Can you work these out from the model? Positions are in its coordinate system, mm. Face numbers are marked on the shaded views. A direction names the side the tool comes from. Round coordinates to 2 decimals unless told otherwise and drop trailing zeros. Order: outer loops, then holes, each group sorted by start corner. A loop starts at its lowest first (then second) coordinate and runs counter-clockwise, first axis right, second up. Notation, with made-up numbers: M 4.5,73 L 39.5,73 A23 ccw 39.5,100 Z; hole C -33,2 d11. An arc over 180 degrees is marked long. Answer as CSV lines item,"result". Start each with the question number.
from build123d import *

# Parameters (mm, degrees)
SKETCH1_R               = 50.8
BOSS_EXTRUDE1_DEPTH     = 101.6
CUT_EXTRUDE1_DEPTH      = 96.52
CUT_EXTRUDE1_DEPTH_BACK = 101.6
SKETCH2_R               = 6.35
CUT_EXTRUDE2_DEPTH      = 103.886
CUT_EXTRUDE2_DEPTH_BACK = 86.36
SKETCH3_W               = 76.2
SKETCH3_H               = 82.476489684


with BuildPart() as part:
    # Sketch1 → Boss-Extrude1 (new body)
    with BuildSketch(Plane(origin=(0, 0, 0), x_dir=(1, 0, 0), z_dir=(0, 1, 0))):
        with Locations(Location((0, 0, 0), (0, 0, 270))):
            Circle(SKETCH1_R)
    extrude(amount=BOSS_EXTRUDE1_DEPTH)

    # Sketch2 → Cut-Extrude1 (cut, two sides: drawn at the far end of the back side and taken through both)
    with BuildSketch(Plane.XY.offset(-CUT_EXTRUDE1_DEPTH_BACK)):
        with Locations(Location((0, 69.85, 0), (0, 0, 180))):
            Circle(SKETCH2_R)
        with BuildLine():
            Line((-50.8, 50.8), (-71.743329605, 50.8))
            Line((-71.743329605, 50.8), (-71.743329605, 136.317810242))
            Line((-71.743329605, 136.317810242), (67.424530317, 136.317810242))
            Line((67.424530317, 136.317810242), (67.424530317, 50.8))
            Line((67.424530317, 50.8), (50.8, 50.8))
            ThreePointArc((50.8, 50.8), (0, 101.6), (-50.8, 50.8))
        make_face()
    extrude(amount=CUT_EXTRUDE1_DEPTH + CUT_EXTRUDE1_DEPTH_BACK, mode=Mode.SUBTRACT)

    # Sketch3 → Cut-Extrude2 (cut, two sides: drawn at the far end of the back side and taken through both)
    with BuildSketch(Plane(origin=(0, 0, 0), x_dir=(0, 0, -1), z_dir=(1, 0, 0)).offset(-CUT_EXTRUDE2_DEPTH_BACK)):
        with Locations((0, 92.038244842)):
            Rectangle(SKETCH3_W, SKETCH3_H)
    extrude(amount=CUT_EXTRUDE2_DEPTH + CUT_EXTRUDE2_DEPTH_BACK, mode=Mode.SUBTRACT)


solid = part.part
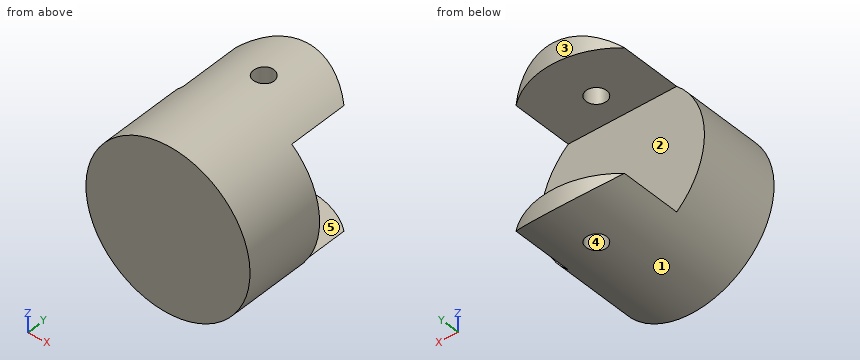
(1) I want a section at A-A on x = 0. Write out the boundary of the cut face in (y, z), and give its area (3 significant figures).
(2) I'm going to push flat-ended pins straight in: P1, Ø3, axis at x = -21.5, z = 13.5, coming from the +Y side; P2, Ø1, axis at x = -20, y = 23.5, coming from the +Z side; P3, Ø4, axis at x = 16, y = 25, coming from the +Z side. Where does each tip first touch, or does it pass through?
(3) I want a section at B-B on y = 67. Write out the boundary of the cut face in (x, z).
(4) I want a section at D-D on x = -25.5. Write out the boundary of the cut face in (y, z).
(5) I want a section at C-C on z = 0. Write out the boundary of the cut face in (x, y).
(6) If I drill on line 1 along Y through (x, z) = (0, -47.5); line 2 along Y through (x, z) = (-33.5, 13); line 3 along X through (y, z) = (69.85, 42), over which ranges is the centre line in solid material (lowest first)?
(7) If we mould it in two halves opening along Y, with no side actions, what happens to the marked faces 3, 4 and 5? For each: +Y half, -Y half, draft (parallel to the pull), parting line (faces both ways), or undercut.
(8) For the marked faces 1 and 2, which set-ups out of +Z, -Z, +X, -X, +Y, -Y let a thin tool reach every point of the face, with its end or its side?
From the geometry:
1,outline,"M 0,-50.8 L 63.5,-50.8 L 63.5,-38.1 L 50.8,-38.1 L 50.8,38.1 L 63.5,38.1 L 63.5,50.8 L 0,50.8 Z; M 76.2,-50.8 L 101.6,-50.8 L 101.6,-38.1 L 76.2,-38.1 Z; M 76.2,38.1 L 101.6,38.1 L 101.6,50.8 L 76.2,50.8 Z"
1,area,"6,130 mm²"
2,P1,"y = 50.8"
2,P2,"z = 46.91"
2,P3,"z = 48.83"
3,outline,"M -33.6,-38.1 A50.8 ccw -5.67,-50.48 L -5.67,-38.1 Z; M -33.6,38.1 L -5.67,38.1 L -5.67,50.48 A50.8 ccw Z; M 5.67,-50.48 A50.8 ccw 33.6,-38.1 L 5.67,-38.1 Z; M 5.67,38.1 L 33.6,38.1 A50.8 ccw 5.67,50.48 Z"
4,outline,"M 0,-43.94 L 94.74,-43.94 L 94.74,-38.1 L 50.8,-38.1 L 50.8,38.1 L 94.74,38.1 L 94.74,43.94 L 0,43.94 Z"
5,outline,"M -50.8,0 L 50.8,0 L 50.8,50.8 L -50.8,50.8 Z"
6,line 1,"0 to 63.5, 76.2 to 101.6"
6,line 2,"0 to 50.8"
6,line 3,"-28.58 to -6.35, 6.35 to 28.58"
7,face 3,"+Y half"
7,face 4,"undercut"
7,face 5,"draft"
8,face 1,"+Y, -Y"
8,face 2,"+X, -X, +Y"
